from build123d import *

# Parameters (mm, degrees)
F1_DEPTH = 12.5
F3_DEPTH = 25
F4_R     = 5


# Not quite as in the source:
# - ends of sketch curves that miss each other by under 0.0002 mm in the source are joined


with BuildPart() as f1:
    # F0 (on Front) → F1 (new body, symmetric)
    with BuildSketch(Plane.XZ):
        with BuildLine():
            Line((-33.4226162893, 0), (33.4226162893, 0))
            Line((33.4226162893, 0), (33.4226162893, 2))
            Line((33.4226162893, 2), (-31.5773837107, 2))
            ThreePointArc((-31.5773837107, 2), (-45.4256059397, 12.9612503934), (-57.4226162893, 0))
            Line((-57.4226162893, 0), (-55.4226162893, 0))
            ThreePointArc((-55.4226162893, 0), (-44.4226162893, 11), (-33.4226162893, 0))
        make_face()
    extrude(amount=F1_DEPTH, both=True)

    # F2 (on face) → F3 (cut)
    with BuildSketch(Plane.XY.offset(2)):
        with BuildLine():
            Line((17.172143635, 2.5), (11.172143635, 2.5))
            ThreePointArc((11.172143635, 2.5), (8.6730891224, -0.0009453085), (11.1740342522, -2.4999998213))
            Line((11.1740342522, -2.4999998213), (17.1730889436, -2.5))
            Line((17.1730889436, -2.5), (17.172143635, 2.5))
        make_face()
        with BuildLine():
            Line((23.172143635, 2.5), (17.172143635, 2.5))
            Line((17.172143635, 2.5), (17.1730889436, -2.5))
            Line((17.1730889436, -2.5), (23.172143635, -2.5))
            ThreePointArc((23.172143635, -2.5), (25.672143635, 0), (23.172143635, 2.5))
        make_face()
        with BuildLine():
            ThreePointArc((-9.3288016735, -2.4999998213), (-6.8278565437, -0.0009453085), (-9.3269110564, 2.4999998213))
            Line((-9.3269110564, 2.4999998213), (-21.3269110564, 2.5))
            ThreePointArc((-21.3269110564, 2.5), (-23.8269110564, 0), (-21.3269110564, -2.5))
            Line((-21.3269110564, -2.5), (-9.3288016735, -2.4999998213))
        make_face()
    extrude(amount=-F3_DEPTH, mode=Mode.SUBTRACT)

    # F4
    f4_edges = [f1.edges().sort_by_distance(p)[0] for p in [
        (33.422616, 12.5, 1),
        (33.422616, -12.5, 1),
        (-56.422616, -12.5, 0),
        (-56.422616, 12.5, 0),
    ]]
    fillet(f4_edges, radius=F4_R)


solid = f1.part
Build history of the part. All positions in model axes, mm. A direction names the side the tool comes from. Round coordinates to 2 decimals unless told otherwise and drop trailing zeros. Loops run counter-clockwise (first coordinate to the right, second up) from the corner with the lowest first, then second, coordinate; pieces in that order, holes last. Notation, with made-up numbers: (-28.75, -18.75) -> (18.25, -18.75) arc R15 cw to (18.25, 7.25) -> close; hole circle Ø2 at (39, -22.75). An arc over 180 degrees is marked (long way). Use CSV: the item, a comma, the result in double quotes. Start each with the question number.
Q1. Flat gauge pins, fed straight in: pin 1 Ø1.5 at (x, z) = (5, 2.5) entering from -Y; pin 2 Ø12 at (x, y) = (-21, 2) entering from +Z; pin 3 Ø2 at (y, z) = (-2, 8.5) entering from +X; pin 4 Ø4 at (y, z) = (-6, 9) entering from -X. Where does each tip first touch, or does it go through?
Q2. Saw through at B-B on x = -19. Give the cut face in (y, z).
Q3. Mould opens along X. For faces 5 (the face through (-17, -12.5, 1)), 6 (the face through (-6.83, -0.06, 1.01)), 7 (the face through (31.919, 11.074, 1.014)), 8 (the face through (-23.826, 0.055, 1.014)) say: +X half, -X half, draft (parallel to the pull), parting line (faces both ways), or undercut.
Q4. Drill centre lines: L1, parallel to Z at x = -2, y = -1; L2, parallel to Z at x = -45, y = 0; L3, parallel to X at y = -2.5, z = 10. Where is each one in solid material? Low to high.
Q5. Saw through at C-C on z = 8. Give the cut face in (x, y).
Q6. Which spindle directions (+Z, -Z, +X, -X, +Y, -Y) get a long thin tool onto all of the face, cutting with end or side? Do faces 1 (the face through (-56.15, -11.07, 1.5)), 2 (the face through (25.67, -0.05, 1.01)), 3 (the face through (-56.15, 11.07, 1.5)), 4 (the face through (1, 0, 2)). Say none if no direction does.
Q7. Saw through at D-D on x = 3. Give the cut face in (y, z), and give its area (3 significant figures).
Q8. Saw through at A-A on y = 0. Give the cut face in (x, z), and give its area (3 significant figures).
Solutions:
1,pin 1,"stops at y = -12.5"
1,pin 2,"stops at z = 2"
1,pin 3,"stops at x = -33.8"
1,pin 4,"stops at x = -55.38"
2,outline,"(-12.5, 0) -> (-2.5, 0) -> (-2.5, 2) -> (-12.5, 2) -> close; (2.5, 0) -> (12.5, 0) -> (12.5, 2) -> (2.5, 2) -> close"
3,face 5,"draft"
3,face 6,"undercut"
3,face 7,"+X half"
3,face 8,"undercut"
4,L1,"z = 0 to 2"
4,L2,"z = 10.98 to 12.99"
4,L3,"x = -52.73 to -49.01, -39.84 to -36.12"
5,outline,"(-54.67, -12.5) -> (-51.97, -12.5) -> (-51.97, 12.5) -> (-54.67, 12.5) -> close; (-36.87, -12.5) -> (-34.18, -12.5) -> (-34.18, 12.5) -> (-36.87, 12.5) -> close"
6,face 1,"-Z, -X, -Y"
6,face 2,"+Z, -Z"
6,face 3,"-Z, -X, +Y"
6,face 4,"+Z, +X, +Y, -Y"
7,outline,"(-12.5, 0) -> (12.5, 0) -> (12.5, 2) -> (-12.5, 2) -> close"
7,area,"50.0 mm^2"
8,outline,"(-57.42, 0) -> (-55.42, 0) arc R11 cw to (-33.42, 0) -> (-23.83, 0) -> (-23.83, 2) -> (-31.58, 2) arc R13 ccw to start; (-6.83, 0) -> (8.67, 0) -> (8.67, 2) -> (-6.83, 2) -> close; (25.67, 0) -> (33.42, 0) -> (33.42, 2) -> (25.67, 2) -> close"
8,area,"137 mm^2"
